Read the model definition and answer for the solid it produces. Units are mm, in the model's axes. Round coordinates to 2 decimals unless told otherwise and drop trailing zeros. Write each loop counter-clockwise with the first axis right and the second up, starting at its lowest first coordinate (ties: lowest second). Pieces come first, ordered by that corner, then holes. Notation, with made-up numbers: (79.25, -29.5) -> (93.25, -29.5) arc R22 cw to (93.25, -7.5) -> close; hole circle Ø7 at (67.5, 1.5). An arc over 180 degrees is marked (long way). Return JSON: item names as keys, results as strings.
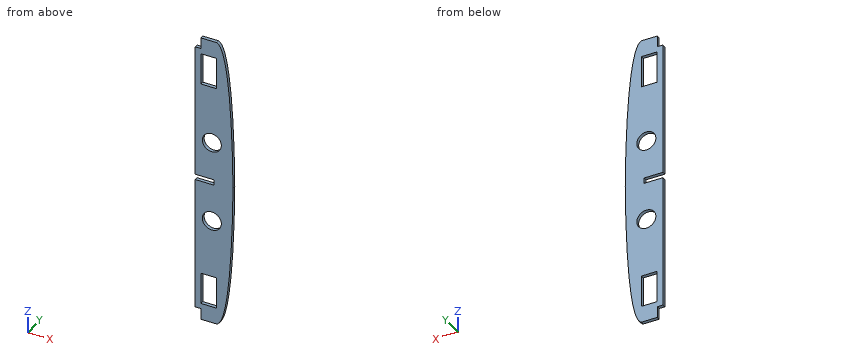
from build123d import *

# Parameters (mm, degrees)
F0_R     = 16.9272487263
F0_W     = 28.0263870955
F0_H     = 56.8133033812
F1_DEPTH = 6


# Not quite as in the source:
# - a feature names something its author has since deleted; it is built from what else it names


with BuildPart() as f1:
    # F0 (on Front) → F1 (new body)
    with BuildSketch(Plane.XZ):
        with BuildLine():
            add(Edge.make_bspline(
                [(181.3542903333, 259), (206.5942975175, 252.0158164026), (209.7991991798, 56.7803677557), (210.2653369369, 6.6428164877)],
                knots=[0, 0, 0, 0, 231.86444259, 231.86444259, 231.86444259, 231.86444259], degree=3))
            Line((181.3542903333, 259), (153.3542903333, 259))
            Line((153.3542903333, 259), (153.3542903333, 239))
            Line((153.3542903333, 239), (143.3542903333, 239))
            Line((143.3542903333, 239), (143.3542903333, 0))
            Line((143.3542903333, 0), (176.8542903333, 0))
            Line((176.8542903333, 0), (176.8542903333, -5))
            Line((176.8542903333, -5), (210.3542903333, -5))
            add(Edge.make_bspline(
                [(210.2653369369, 6.6428164877), (210.3331344644, -0.6494527163), (210.3429952934, -4.8722740171), (210.3542903333, -5)],
                knots=[231.86444259, 231.86444259, 231.86444259, 231.86444259, 265.5880268386, 265.5880268386, 265.5880268386, 265.5880268386], degree=3))
        make_face()
        with Locations((172.8220252337, 68.3807536824)):
            Circle(F0_R, mode=Mode.SUBTRACT)
        with Locations((167.491195113, 200.8973438895)):
            Rectangle(F0_W, F0_H, mode=Mode.SUBTRACT)
        with BuildLine():
            add(Edge.make_bspline(
                [(210.2653369369, -16.6428164877), (210.3331344644, -9.3505472837), (210.3429952934, -5.1277259829), (210.3542903333, -5)],
                knots=[231.86444259, 231.86444259, 231.86444259, 231.86444259, 265.5880268386, 265.5880268386, 265.5880268386, 265.5880268386], degree=3))
            Line((210.3542903333, -5), (176.8542903333, -5))
            Line((176.8542903333, -5), (176.8542903333, -10))
            Line((176.8542903333, -10), (143.3542903333, -10))
            Line((143.3542903333, -10), (143.3542903333, -249))
            Line((143.3542903333, -249), (153.3542903333, -249))
            Line((153.3542903333, -249), (153.3542903333, -269))
            Line((153.3542903333, -269), (181.3542903333, -269))
            add(Edge.make_bspline(
                [(181.3542903333, -269), (206.5942975175, -262.0158164026), (209.7991991798, -66.7803677557), (210.2653369369, -16.6428164877)],
                knots=[0, 0, 0, 0, 231.86444259, 231.86444259, 231.86444259, 231.86444259], degree=3))
        make_face()
        with Locations((167.491195113, -210.8973438895)):
            Rectangle(F0_W, F0_H, mode=Mode.SUBTRACT)
        with Locations((172.8220252337, -78.3807536824)):
            Circle(F0_R, mode=Mode.SUBTRACT)
    extrude(amount=F1_DEPTH)


solid = f1.part
Item 1: Section B-B (y = -3) is taken. State how many separate pieces and enclosed holes the cut face has, then the cut area to 3 significant figures.
Worked answers:
{"separate pieces": "1", "enclosed holes": "4", "area": "26,400 mm2"}
Item 2: Straight lines are drawn through the part: L1, parallel to Z at x = 154.5, y = -1.5; L2, parallel to Z at x = 174.5, y = -3.75; L3, parallel to Z at x = 183.5, y = -3.75. For each, find the intervals that lie inside material, in ascending order. Write a range as [from, to].
Worked answers:
{"L1": "z = [-269, -239.3], [-182.49, -10], [0, 172.49], [229.3, 259]", "L2": "z = [-269, -239.3], [-182.49, -95.22], [-61.54, -10], [0, 51.54], [85.22, 172.49], [229.3, 259]", "L3": "z = [-267.92, -91.52], [-65.25, 55.25], [81.52, 257.92]"}
Item 3: Flat-ended cylindrical pins translate along their axes: pin 1 (1.8 mm diameter, centred on x = 149.5, y = -3, fed in from +Z); pin 2 (2 mm diameter, centred on x = 150.5, y = -3.5, fed in from -Z); pin 3 (1.8 mm diameter, centred on y = -3, z = -3.5, fed in from -X). Find the tip coordinate at first contact, or state that the pin passes through.
Worked answers:
{"pin 1": "stops at z = 239", "pin 2": "stops at z = -249", "pin 3": "stops at x = 176.85"}
Item 4: Section A-A (x = 148.5) is taken. Give the vertices of the cut face in (y, z), then the cut area to 3 significant figures.
Worked answers:
{"outline": "(-6, -249) -> (0, -249) -> (0, -10) -> (-6, -10) -> close; (-6, 0) -> (0, 0) -> (0, 239) -> (-6, 239) -> close", "area": "2,870 mm2"}
